The model under review builds one solid part; all positions refer to its coordinate system, in mm. Face numbers are marked on the shaded views. A direction names the side the tool comes from. Round coordinates to 2 decimals unless told otherwise and drop trailing zeros. Write each loop counter-clockwise with the first axis right and the second up, starting at its lowest first coordinate (ties: lowest second). Pieces come first, ordered by that corner, then holes. Notation, with made-up numbers: (74, 54.5) - (110, 54.5) arc R19 cw to (110, 91.5) - close; hole circle Ø3 at (66.5, 39.25). An arc over 180 degrees is marked (long way). Write each question's results on one line, items separated by ' | '.
Autodesk Inventor part; units mm, degrees
ref_plane "YZ Plane" through (0, 0, 0) normal (1, 0, 0) x (0, 1, 0)
ref_plane "XZ Plane" through (0, 0, 0) normal (0, 1, 0) x (-1, 0, 0)
ref_plane "XY Plane" through (0, 0, 0) normal (0, 0, 1) x (1, 0, 0)
sketch "Sketch1" plane through (0, 0, 0) normal (0, 0, 1) x (1, 0, 0)
  line L0 (5.3975, 5.374) -> (29.8975, 5.374)
  line L1 (5.3975, 27.374) -> (29.8975, 27.374)
  line L2 (5.3975, 5.374) -> (5.3975, 27.374)
  arc A0 (29.8975, 20.874) -> (29.8975, 11.874) centre (29.8975, 16.374) ccw
  line L3 (29.8975, 20.874) -> (39.9349, 20.874)
  line L4 (29.8975, 11.874) -> (39.9349, 11.874)
  arc A1 (29.8975, 5.374) -> (39.9349, 11.874) centre (29.8975, 16.374) ccw
  arc A2 (39.9349, 20.874) -> (29.8975, 27.374) centre (29.8975, 16.374) ccw
  point P0 (0, 0)
  dimension "d0" = 9
extrude "Extrusion1" add sketch "Sketch1" along normal blind 47
sketch "Sketch2" plane through (5.3975, 5.374, 0) normal (0, -1, 0) x (1, 0, 0)
  line L0 (24.5, 47) -> (0, 47)
  line L1 (0, 0) -> (0, 47)
  line L2 (24.5, 0) -> (24.5, 47)
  line L3 (3, 44) -> (34.5374, 44)
  line L4 (34.5374, 0) -> (34.5374, 47)
  line L5 (34.5374, 44) -> (34.5374, 3)
  line L6 (3, 44) -> (3, 3)
  line L7 (3, 3) -> (34.5374, 3)
  line L8 (34.5374, 0) -> (24.5, 0)
  point P0 (-5.3975, 0)
  dimension "d3" = 3
  dimension "d4" = 3
  dimension "d5" = 3
extrude "Extrusion2" cut sketch "Sketch2" against normal through all contours L7 L6 L3 L2 | L2 L3 L4 L7
sketch "Sketch3" plane through (5.3975, 5.374, 0) normal (-1, 0, 0) x (0, 0, 1)
  circle A0 centre (23.5, 11) radius 4.5
  point P0 (0, -5.374)
  dimension "d8" = 9
extrude "Extrusion3" cut sketch "Sketch3" against normal through all
sketch "Sketch4" plane through (0, 0, 0) normal (0, 0, -1) x (-1, 0, 0)
  line L0 (-5.3975, 5.374) -> (-29.8975, 5.374)
  arc A0 (-29.8975, 27.374) -> (-39.9349, 20.874) centre (-29.8975, 16.374) ccw
  arc A1 (-29.8975, 11.874) -> (-29.8975, 20.874) centre (-29.8975, 16.374) ccw
  arc A2 (-39.9349, 11.874) -> (-29.8975, 5.374) centre (-29.8975, 16.374) ccw
  circle A3 centre (-22.0445, 19.6268) radius 1
  line L1 (-29.8975, 16.374) -> (-22.0445, 19.6268)
  circle A4 centre (-26.6447, 24.2269) radius 1
  circle A5 centre (-33.1503, 24.2269) radius 1
  circle A6 centre (-37.7505, 19.6268) radius 1
  circle A7 centre (-37.7505, 13.1211) radius 1
  circle A8 centre (-33.1503, 8.521) radius 1
  circle A9 centre (-26.6447, 8.521) radius 1
  circle A10 centre (-22.0445, 13.1211) radius 1
  point P0 (0, 0)
  dimension "d11" = 2
  dimension "d12" = 8.5
  dimension "d13" = 22.5
  dimension "d16" = 360
extrude "Extrusion4" cut sketch "Sketch4" against normal through all contours A3 | A4 | A5 | A8 | A9 | A10
sketch "Sketch5" plane through (8.3975, 5.374, 44) normal (1, 0, 0) x (0, 0, -1)
  circle A0 centre (20.5, 11) radius 4.5
  circle A1 centre (20.5, 19.5) radius 1
  point P0 (44, -5.374)
  dimension "d20" = 2
  dimension "d21" = 8.5
extrude "Extrusion5" cut sketch "Sketch5" against normal through all contours A1
pattern_circular "Circular Pattern1" count 8 over 360 about axis through (5.3975, 16.374, 23.5) along (1, 0, 0) of "Extrusion5"
properties part number "Shoulder" material "Aluminum-6061"
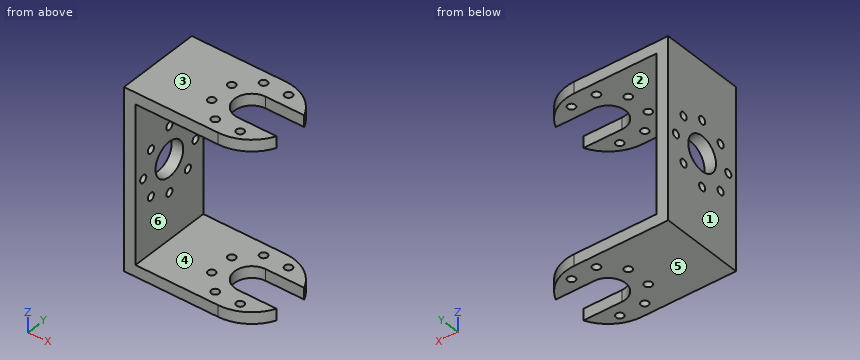
Q1. For probe 1 along Y at (x, z) = (6.65, 23.5); probe 2 along Z at (x, y) = (26, 19.25); probe 3 along Z at (x, y) = (8, 25), list the stretches that pass through material, from the lowest coordinate up.
Evaluation:
probe 1: y = 5.37 to 6.87, 8.87 to 11.87, 20.87 to 23.87, 25.87 to 27.37 | probe 2: z = 0 to 3, 44 to 47 | probe 3: z = 0 to 22.51, 24.49 to 47
Q2. Tool access review of the marked faces 1 and 2: name each direction out of +Z, -Z, +X, -X, +Y, -Y from which nothing blocks a thin tool from reaching the whole face with its end or side.
Evaluation:
face 1: +Z, -Z, -X, +Y, -Y | face 2: +X, +Y, -Y
Q3. We need section A-A (z = 23.5). State the section outline as (x, y) points.
Evaluation:
outline: (5.4, 5.37) - (8.4, 5.37) - (8.4, 6.87) - (5.4, 6.87) - close; (5.4, 8.87) - (8.4, 8.87) - (8.4, 11.87) - (5.4, 11.87) - close; (5.4, 20.87) - (8.4, 20.87) - (8.4, 23.87) - (5.4, 23.87) - close; (5.4, 25.87) - (8.4, 25.87) - (8.4, 27.37) - (5.4, 27.37) - close
Q4. We need section C-C (z = 32). State the section outline as (x, y) points.
Evaluation:
outline: (5.4, 5.37) - (8.4, 5.37) - (8.4, 15.37) - (5.4, 15.37) - close; (5.4, 17.37) - (8.4, 17.37) - (8.4, 27.37) - (5.4, 27.37) - close
Q5. We need section B-B (x = 12). State the section outline as (y, z) points.
Evaluation:
outline: (5.37, 0) - (27.37, 0) - (27.37, 3) - (5.37, 3) - close; (5.37, 44) - (27.37, 44) - (27.37, 47) - (5.37, 47) - close
Q6. Insertion check: P1, Ø1.2, axis at x = 22.04, y = 19.63, coming from the +Z side; P2, Ø8, axis at y = 19.5, z = 30, coming from the +X side; P3, Ø1.5, axis at x = 34.5, z = 46, coming from the -Y side; P4, Ø0.9, axis at x = 35, z = 1, coming from the -Y side. Each pin has a flat end and moves straight along its axis. Give the tip position at first contact, or say it passes through.
Evaluation:
P1: passes through | P2: stops at x = 8.4 | P3: stops at y = 6.07 | P4: stops at y = 6.41
Q7. We need section D-D (x = 22.5). State the section outline as (y, z) points, plus the area to 3 significant figures.
Evaluation:
outline: (5.37, 0) - (12.23, 0) - (12.23, 3) - (5.37, 3) - close; (5.37, 44) - (12.23, 44) - (12.23, 47) - (5.37, 47) - close; (14.01, 0) - (18.74, 0) - (18.74, 3) - (14.01, 3) - close; (14.01, 44) - (18.74, 44) - (18.74, 47) - (14.01, 47) - close; (20.52, 0) - (27.37, 0) - (27.37, 3) - (20.52, 3) - close; (20.52, 44) - (27.37, 44) - (27.37, 47) - (20.52, 47) - close | area: 111 mm^2
Q8. The part is to be moulded in two halves that separate along Z. For the marked faces 3, 4, 5 and 6, say which applies: released by +Z, released by -Z, zero draft, split by the parting line, or undercut.
Evaluation:
face 3: released by +Z | face 4: undercut | face 5: released by -Z | face 6: undercut
